Build history of the part. All positions in model axes, mm. A direction names the side the tool comes from. Round coordinates to 2 decimals unless told otherwise and drop trailing zeros. Order: outer loops, then holes, each group sorted by start corner. A loop starts at its lowest first (then second) coordinate and runs counter-clockwise, first axis right, second up. Notation, with made-up numbers: M 27.5,-6.5 L 42.5,-6.5 A19 cw 42.5,21.5 Z; hole C 27.5,-34.5 d6. An arc over 180 degrees is marked long. Use CSV: the item, a comma, the result in double quotes.
from build123d import *

# Parameters (mm, degrees)
F0_W     = 114.3
F0_H     = 88.9
F1_DEPTH = 25.4
F3_DEPTH = 25.4
F4_R     = 19.164267
F5_DEPTH = 50.8


with BuildPart() as f1:
    # F0 (on Front) → F1 (new body)
    with BuildSketch(Plane.XZ):
        with Locations((-16.952309, -7.416258)):
            Rectangle(F0_W, F0_H)
    extrude(amount=-F1_DEPTH)

    # F2 (on Front) → F3 (join)
    with BuildSketch(Plane.XZ):
        Polygon((17.68492, -51.485937), (-40.78941, 37.509143), (-73.592082, 37.509143), (-73.592082, -51.485937), align=None)
    extrude(amount=F3_DEPTH)

    # F4 (on Front) → F5 (cut)
    with BuildSketch(Plane.XZ):
        with Locations((-24.245456, 10.696524)):
            Circle(F4_R)
    extrude(amount=-F5_DEPTH, mode=Mode.SUBTRACT)


solid = f1.part
(1) Wall check: line 1 (Z direction, x = 9.5, y = 2); line 2 (Y direction, x = -17, z = 29.5); line 3 (X direction, y = 14, z = 17.5). Give the ranges that are in metal, low to high. Write a range as from..to.
Answer block:
line 1,"z = -51.87..37.03"
line 2,"y = 0..25.4"
line 3,"x = -74.1..-42.16, -6.33..40.2"
(2) Cut at A-A, the plane x = -26.5. Give the cut face in (y, z).
Answer block:
outline,"M -25.4,-51.49 L 0,-51.49 L 0,-51.87 L 25.4,-51.87 L 25.4,-8.33 L 0,-8.33 L 0,15.76 L -25.4,15.76 Z; M 0,29.73 L 25.4,29.73 L 25.4,37.03 L 0,37.03 Z"
(3) Two-plate mould, pull along Y, no slides. Class faces 5 (the face through (-18, 13, 37.034)), 6 (the face through (-32, 0, 6)), 7 (the face through (-39, -25.4, -16)): released by +Y, released by -Y, zero draft, split by the parting line, or undercut.
Answer block:
face 5,"zero draft"
face 6,"released by +Y"
face 7,"released by -Y"
(4) Drop flat-ended pins along their axis: pin 1 (23 mm diameter, centred on x = -24.25, z = 10.7, fed in from +Y); pin 2 (3 mm diameter, centred on y = -5.5, z = -39, fed in from -X); pin 3 (10 mm diameter, centred on y = -0.5, z = 20.5, fed in from +X); pin 4 (1.5 mm diameter, centred on x = 6.5, y = 5, fed in from +Z). Give the stop position or say it passes through.
Answer block:
pin 1,"stops at y = 0"
pin 2,"stops at x = -73.59"
pin 3,"stops at x = 40.2"
pin 4,"stops at z = 37.03"
(5) Cut at B-B, the plane z = -14. Give the cut face in (x, y).
Answer block:
outline,"M -74.1,0 L -73.59,0 L -73.59,-25.4 L -6.95,-25.4 L -6.95,0 L 40.2,0 L 40.2,25.4 L -74.1,25.4 Z"
(6) Tool access for faces 1 (the face through (-39.454, 12.522, -0.965)), 2 (the face through (-73.592, -13, -6)), 3 (the face through (-11.143, -12.522, -7.611)), 4 (the face through (-29, -13, -51.486)): list every direction of +Z, -Z, +X, -X, +Y, -Y with a clear straight run to the whole face (end or side of a thin tool).
Answer block:
face 1,"+Y"
face 2,"+Z, -Z, -X, -Y"
face 3,"+Z, +X, -Y"
face 4,"-Z, +X, -X, -Y"
(7) Cut at D-D, the plane y = -14.5. Give the cut face in (x, z), and give its area (3 significant figures).
Answer block:
outline,"M -73.59,-51.49 L 17.68,-51.49 L -40.79,37.51 L -73.59,37.51 Z"
area,"5,520 mm²"
(8) Cut at C-C, the plane z = 21. Give the cut face in (x, y).
Answer block:
outline,"M -74.1,0 L -73.59,0 L -73.59,-25.4 L -29.94,-25.4 L -29.94,0 L -40.4,0 L -40.4,25.4 L -74.1,25.4 Z; M -8.09,0 L 40.2,0 L 40.2,25.4 L -8.09,25.4 Z"
